from build123d import *

# Parameters (mm, degrees)
SKETCH1_R           = 2.5
BOSS_EXTRUDE1_DEPTH = 3
FILLET1_R           = 2


with BuildPart() as part:
    # Sketch1 → Boss-Extrude1 (new body)
    with BuildSketch(Plane(origin=(0, 0, 0), x_dir=(0, 0, -1), z_dir=(1, 0, 0))):
        Polygon((75, 0), (0, 0), (0, 75), (20, 75), (75, 20), align=None)
        with Locations((65, 10)):
            Circle(SKETCH1_R, mode=Mode.SUBTRACT)
        with Locations((37.5, 10)):
            Circle(SKETCH1_R, mode=Mode.SUBTRACT)
        with Locations((10, 10)):
            Circle(SKETCH1_R, mode=Mode.SUBTRACT)
        with Locations((10, 65)):
            Circle(SKETCH1_R, mode=Mode.SUBTRACT)
        with Locations((10, 37.5)):
            Circle(SKETCH1_R, mode=Mode.SUBTRACT)
    extrude(amount=BOSS_EXTRUDE1_DEPTH)

    # Fillet1
    fillet1_edges = [part.edges().sort_by_distance(p)[0] for p in [
        (1.5, 0, -75),
        (1.5, 0, 0),
        (1.5, 75, 0),
        (1.5, 75, -20),
        (1.5, 20, -75),
    ]]
    fillet(fillet1_edges, radius=FILLET1_R)


solid = part.part
Verification items for the finished model (mm, model axes). Give positions to 0.01 mm unless a question says otherwise; leave off trailing zeros. Write each loop counter-clockwise with the first axis right and the second up, starting at its lowest first coordinate (ties: lowest second). Pieces come first, ordered by that corner, then holes.
(1) Mould release check, pull along Z, two halves, no side actions. Record for faces 1 (the face through (1, 37, 0)), 2 (the face through (1.48, 7.56, -9.46)), 3 (the face through (3, 30, -30)): +Z half, -Z half, draft (parallel to the pull), parting line (faces both ways), or undercut.
(2) Cross-section at D-D (z = -10). Enter the section's corners in (x, y).
(3) Material ranges on line 1 (Y direction, x = 1, z = -10); line 2 (Z direction, x = 2.1, y = 60); line 3 (Y direction, x = 0.85, z = -11.5), recorded low to high.
(4) Gauge pin test, flat end, axial feed: pin 1 (4 mm diameter, centred on y = 62, z = -29, fed in from -X). Record the tip position at first contact, or that the pin passes through.
(5) Cross-section at A-A (z = -65). Enter the section's corners in (x, y).
(6) Cross-section at B-B (y = 65). Enter the section's corners in (x, z).
(7) Cross-section at C-C (x = 2.45). Enter the section's corners in (y, z).
Worked out:
1. face 1: +Z half
1. face 2: undercut
1. face 3: draft
2. outline: (0, 0) - (3, 0) - (3, 7.5) - (0, 7.5) - close; (0, 12.5) - (3, 12.5) - (3, 35) - (0, 35) - close; (0, 40) - (3, 40) - (3, 62.5) - (0, 62.5) - close; (0, 67.5) - (3, 67.5) - (3, 75) - (0, 75) - close
3. line 1: y = 0 to 7.5, 12.5 to 35, 40 to 62.5, 67.5 to 75
3. line 2: z = -35 to 0
3. line 3: y = 0 to 8, 12 to 35.5, 39.5 to 63, 67 to 75
4. pin 1: stops at x = 0
5. outline: (0, 0) - (3, 0) - (3, 7.5) - (0, 7.5) - close; (0, 12.5) - (3, 12.5) - (3, 30) - (0, 30) - close
6. outline: (0, -30) - (3, -30) - (3, -12.5) - (0, -12.5) - close; (0, -7.5) - (3, -7.5) - (3, 0) - (0, 0) - close
7. outline: (0, -73) arc R2 ccw to (2, -75) - (19.17, -75) arc R2 ccw to (20.59, -74.41) - (74.41, -20.59) arc R2 ccw to (75, -19.17) - (75, -2) arc R2 ccw to (73, 0) - (2, 0) arc R2 ccw to (0, -2) - close; hole circle Ø5 at (10, -65); hole circle Ø5 at (10, -37.5); hole circle Ø5 at (10, -10); hole circle Ø5 at (37.5, -10); hole circle Ø5 at (65, -10)
